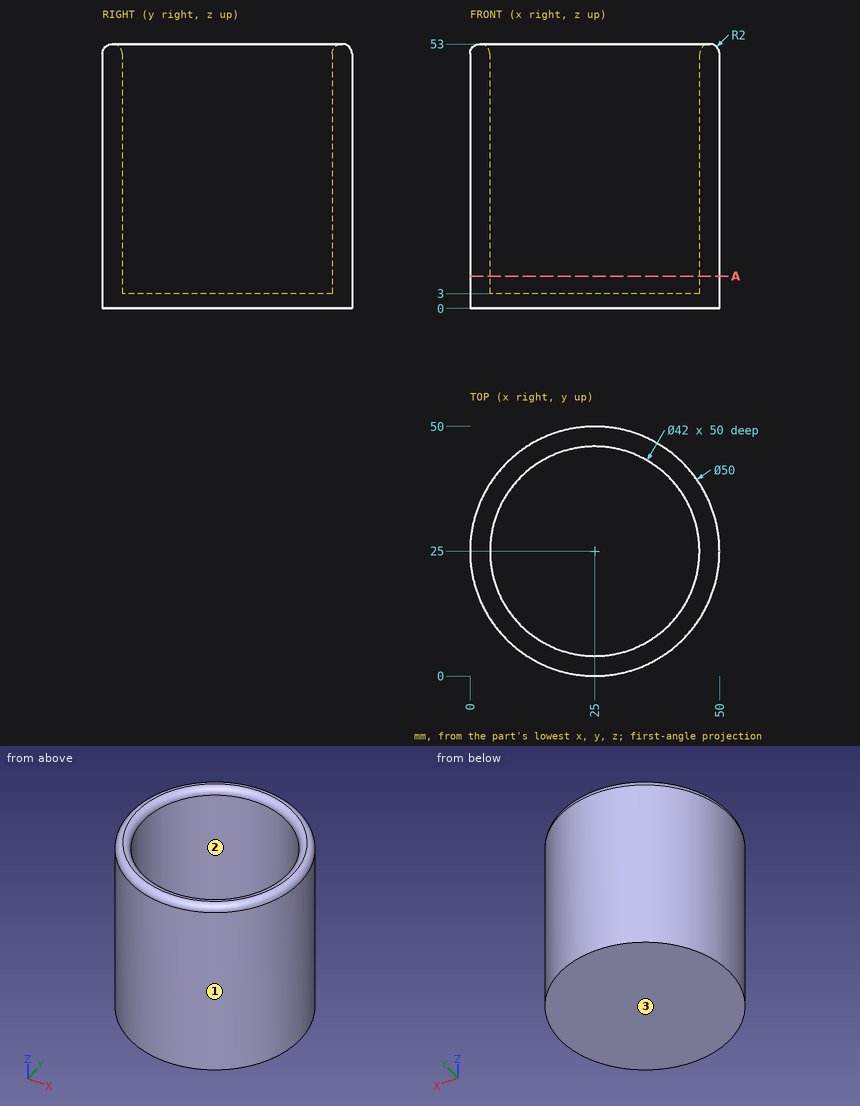
Check sheet for the drawn part. Datum: minimum x, y, z corner. Units: mm. Give positions to 0.01 mm unless a question says otherwise; leave off trailing zeros. Order: outer loops, then holes, each group sorted by start corner. A loop starts at its lowest first (then second) coordinate and runs counter-clockwise, first axis right, second up. Notation, with made-up numbers: (43.5, 59.25) - (93.5, 59.25) arc R30 cw to (93.5, 87.25) - close; hole circle Ø10 at (-38, 81.5). An arc over 180 degrees is marked (long way). Answer as a JSON object with one key per item and string values.
(1) Material ranges on line 1 (Y direction, x = 25, z = 40); line 2 (Z direction, x = 33, y = 44); line 3 (X direction, y = 26, z = 44), recorded low to high.
Report:
{"line 1": "0 to 4, 46 to 50", "line 2": "0 to 3", "line 3": "0.02 to 4.02, 45.98 to 49.98"}
(2) Draft check along X on the marked faces 1, 2 and 3. Enter one of: released by +X, released by -X, zero draft, split by the parting line, or undercut.
Report:
{"face 1": "split by the parting line", "face 2": "undercut", "face 3": "zero draft"}
(3) Cross-section at A-A (z = 6.5). Record the cut outline in (x, y), then the cut area to 3 significant figures.
Report:
{"outline": "circle Ø50 at (25, 25); hole circle Ø42 at (25, 25)", "area": "578 mm^2"}
(4) Depth check by flat-ended pin: pin 1 Ø4 at (y, z) = (30, 34.5) entering from -X; pin 2 Ø4 at (y, z) = (15, 27.5) entering from -X; pin 3 Ø5 at (y, z) = (17, 47.5) entering from -X. Enter the tip coordinate at first touch or a pass-through.
Report:
{"pin 1": "x = 0.18", "pin 2": "x = 1.31", "pin 3": "x = 0.61"}
